Can you work these out from the model? Positions are in its coordinate system, mm. A direction names the side the tool comes from. Coordinates: 2 decimals unless noted, no trailing zeros. Write each loop counter-clockwise with the first axis right and the second up, starting at its lowest first coordinate (ties: lowest second). Pieces come first, ordered by that corner, then holes. Notation, with made-up numbers: M 30.25,52.25 L 40.25,52.25 A24 ccw 40.25,68.25 Z; hole C 28,-36.75 d6. An arc over 180 degrees is marked long. Use one line per item in the form item = value. Start each with the question number.
```python
from build123d import *

# Parameters (mm, degrees)
F2_DEPTH      = 8
F2_DEPTH_BACK = 8
F3_R          = 3


# Not quite as in the source:
# - two fillets or chamfers of one size are made in one step


with BuildPart() as f2:
    # F1 (on Top) → F2 (new body, two sides)
    with BuildSketch(Plane.XY) as f2_sk:
        Polygon((-55, -8), (-50, -8), (-50, 8), (-50, 18), (-55, 18), align=None)
        Polygon((-50, -8), (30.9022613208, -8), (50, -6.0806050441), (50, 8), (-50, 8), align=None)
        Polygon((50, 8), (50, -6.0806050441), (53, -5.7790936996), (53, 10), (50, 10), align=None)
    extrude(amount=F2_DEPTH)
    extrude(f2_sk.sketch, amount=-F2_DEPTH_BACK)

    # F3 (call 1 of 7: OpenCascade refuses the feature's edges together)
    f3_edges = [f2.edges().sort_by_distance(p)[0] for p in [
        (-12.048869, -8, 8),
        (-55, -8, 0),
        (30.902261, -8, 0),
        (-12.048869, -8, -8),
        (41.951131, -6.889547, 8),
        (41.951131, -6.889547, -8),
    ]]
    fillet(f3_edges, radius=F3_R)

    # F3#2 (call 2 of 7)
    f3_2_edges = [f2.edges().sort_by_distance(p)[0] for p in [
        (-52.5, 18, -8),
    ]]
    fillet(f3_2_edges, radius=F3_R)

    # F3#3 (call 3 of 7)
    f3_3_edges = [f2.edges().sort_by_distance(p)[0] for p in [
        (-52.5, 18, 8),
    ]]
    fillet(f3_3_edges, radius=F3_R)

    # F3#4 (call 4 of 7)
    f3_4_edges = [f2.edges().sort_by_distance(p)[0] for p in [
        (0, 8, 8),
    ]]
    fillet(f3_4_edges, radius=F3_R)

    # F3#5 (call 5 of 7)
    f3_5_edges = [f2.edges().sort_by_distance(p)[0] for p in [
        (0, 8, -8),
    ]]
    fillet(f3_5_edges, radius=F3_R)

    # F3#6 (call 6 of 7)
    f3_6_edges = [f2.edges().sort_by_distance(p)[0] for p in [
        (51.5, 10, -8),
    ]]
    fillet(f3_6_edges, radius=F3_R)

    # F3#7 (call 7 of 7)
    f3_7_edges = [f2.edges().sort_by_distance(p)[0] for p in [
        (51.5, 10, 8),
    ]]
    fillet(f3_7_edges, radius=F3_R)


solid = f2.part
```
1) Please list where these lines run through material, in increasing order: line 1 (X direction, y = 9.75, z = 2); line 2 (Y direction, x = 13.5, z = 2); line 3 (X direction, y = 14.25, z = 0.5).
2) If we mould it in two halves opening along X, with no side actions, what happens to faces 1 (the face through (-54.1, -7.14, -0.11)), 2 (the face through (-50, 13, 0)), 3 (the face through (52, 10, 0)), 4 (the face through (53, 2, 0))? For each: +X half, -X half, draft (parallel to the pull), parting line (faces both ways), or undercut.
3) Suppose I cut it at C-C on y = 12. Please give me the cut outline in (x, z).
4) Will these pins go through, and if not, where does the flat tip stop? pin 1 Ø5 at (x, z) = (6.5, 1) entering from +Y; pin 2 Ø4 at (y, z) = (13, -0.5) entering from +X; pin 3 Ø1.5 at (x, z) = (52, -1) entering from +Y.
5) Suppose I cut it at B-B on z = -1.5. Please give me the cut outline in (x, y).
6) Which directions (+Z, -Z, +X, -X, +Y, -Y) give clear straight access to the entire face, cutting with the end or side of a thin tool? Please do faces 5 (the face through (-0.7, 7.1, 7.14)), 6 (the face through (51.48, 9.1, -7.14)), 7 (the face through (51.48, 9.14, 7.1)).
7) Suppose I cut it at D-D on z = -6.5. Please give me the cut outline in (x, y), and give its area (3 significant figures).
8) Suppose I cut it at A-A on x = 3. Please give me the cut outline in (y, z).
Computed values:
q1.line_1 = -55 to -50, 50 to 53
q1.line_2 = -8 to 8
q1.line_3 = -55 to -50
q2.face_1 = -X half
q2.face_2 = undercut
q2.face_3 = draft
q2.face_4 = +X half
q3.outline = M -55,-8 L -50,-8 L -50,8 L -55,8 Z
q4.pin_1 = 8
q4.pin_2 = -50
q4.pin_3 = 10
q5.outline = M -55,-5 A3 ccw -52,-8 L 30.75,-8 A3 ccw 31.05,-7.98 L 53,-5.78 L 53,10 L 50,10 L 50,8 L -50,8 L -50,18 L -55,18 Z
q6.face_5 = +Z, +Y
q6.face_6 = -Z, +X, +Y
q6.face_7 = +Z, +X, +Y
q7.outline = M -55,-5 A3 ccw -53.5,-7.6 L 30.75,-7.6 A2.6 ccw 31.01,-7.59 L 53,-5.38 L 53,9.6 L 50,9.6 L 50,7.6 L -50,7.6 L -50,17.6 L -55,17.6 Z
q7.area = 1,670 mm²
q8.outline = M -8,-5 A3 ccw -5,-8 L 5,-8 A3 ccw 8,-5 L 8,5 A3 ccw 5,8 L -5,8 A3 ccw -8,5 Z
